Can you work these out from the model? Positions are in its coordinate system, mm. Give positions to 0.01 mm unless a question says otherwise; leave off trailing zeros. Loops run counter-clockwise (first coordinate to the right, second up) from the corner with the lowest first, then second, coordinate; pieces in that order, holes last. Notation, with made-up numbers: (39.5, 72.5) - (67.5, 72.5) arc R21 cw to (67.5, 106.5) - close; hole circle Ø1 at (5.25, 71). An arc over 180 degrees is marked (long way). Answer as a JSON object with one key per item and string values. Group by question number.
Item 1: Suppose I cut it at A-A on x = 69. Write out the boundary of the cut face in (y, z), and give its area (3 significant figures).
Item 2: Please list where these lines run through material, in increasing order: L1, parallel to Y at x = 108, z = 0.5; L2, parallel to Y at x = 56, z = 5.75; L3, parallel to Z at x = 112, y = -50.
Item 3: Will these pins go through, and if not, where does the flat tip stop? pin 1 (1.5 mm diameter, centred on y = -25.5, z = 8, fed in from +X); pin 2 (1 mm diameter, centred on x = 56.5, y = -18, fed in from -Z); pin 3 (1.1 mm diameter, centred on y = -78, z = 5.5, fed in from -X).
Item 4: Suppose I cut it at B-B on z = 7.5. Write out the boundary of the cut face in (x, y), and give its area (3 significant figures).
Item 5: Suppose I cut it at C-C on y = -52. Write out the boundary of the cut face in (x, z).
Item 6: Suppose I cut it at D-D on y = -10.5. Write out the boundary of the cut face in (x, z).
from build123d import *

# Parameters (mm, degrees)
BOSS_EXTRUDE1_DEPTH = 10
SKETCH4_W           = 80
SKETCH4_H           = 5
CUT_EXTRUDE1_DEPTH  = 6
SKETCH5_W           = 80
SKETCH5_H           = 80
BOSS_EXTRUDE3_DEPTH = 1


with BuildPart() as part:
    # Sketch1 → Boss-Extrude1 (new body)
    with BuildSketch(Plane.XY):
        Polygon((0, 0), (0, -27), (127, -27), (127, -24), (3, -24), (3, 0), align=None)
    extrude(amount=BOSS_EXTRUDE1_DEPTH)

    # Sketch4 → Cut-Extrude1 (cut)
    with BuildSketch(Plane(origin=(0, -24, 0), x_dir=(1, 0, 0), z_dir=(0, 1, 0))):
        with Locations((87, -7.5)):
            Rectangle(SKETCH4_W, SKETCH4_H)
    extrude(amount=-CUT_EXTRUDE1_DEPTH, mode=Mode.SUBTRACT)

    # Sketch5 → Boss-Extrude3 (add)
    with BuildSketch(Plane.XY.offset(5)):
        with Locations((87, -56.52)):
            Rectangle(SKETCH5_W, SKETCH5_H)
    extrude(amount=BOSS_EXTRUDE3_DEPTH)


solid = part.part
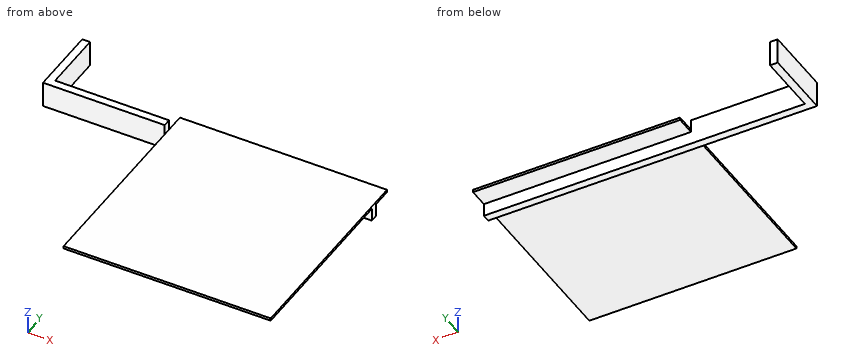
Worked out:
{
 "1": {"outline": "(-96.52, 5) - (-27, 5) - (-27, 0) - (-24, 0) - (-24, 5) - (-16.52, 5) - (-16.52, 6) - (-96.52, 6) - close", "area": "95.0 mm2"},
 "2": {"L1": "y = -27 to -24", "L2": "y = -96.52 to -16.52", "L3": "z = 5 to 6"},
 "3": {"pin 1": "stops at x = 47", "pin 2": "stops at z = 5", "pin 3": "stops at x = 47"},
 "4": {"outline": "(0, -27) - (47, -27) - (47, -24) - (3, -24) - (3, 0) - (0, 0) - close", "area": "213 mm2"},
 "5": {"outline": "(47, 5) - (127, 5) - (127, 6) - (47, 6) - close"},
 "6": {"outline": "(0, 0) - (3, 0) - (3, 10) - (0, 10) - close"}
}
